Work out the finished part from the listing and answer in its coordinate system (mm). Give positions to 0.01 mm unless a question says otherwise; leave off trailing zeros. Write each loop counter-clockwise with the first axis right and the second up, starting at its lowest first coordinate (ties: lowest second). Pieces come first, ordered by that corner, then holes. Notation, with made-up numbers: (65.5, -24.5) -> (78.5, -24.5) arc R35 cw to (78.5, 14.5) -> close; hole circle Ø6 at (50, 18). An arc over 180 degrees is marked (long way). Use a Markdown table: item, result. Add a question column.
Q1. Consider line 1 (Y direction, x = -174, z = 11.5); line 2 (Y direction, x = 0, z = 12.25); line 3 (Y direction, x = 46.5, z = 1.75). Determine where each line is inside the solid, lowest interval first.
Q2. Section C-C, the plane y = -147.5 is taken. Give the vertices of the cut face in (x, z).
Q3. Each of these flat-tipped pins is pushed along its axis until it touches: pin 1 Ø15 at (x, y) = (174, -174) entering from +Z; pin 2 Ø10 at (x, z) = (-36.5, 16) entering from +Y; pin 3 Ø10 at (x, z) = (-15.5, 12) entering from +Y; pin 4 Ø1.5 at (x, z) = (165.5, 7.5) entering from -Y. Where does it stop, or does it pass through?
Q4. Section D-D, the plane y = -12 is taken. Give the vertices of the cut face in (x, z).
Q5. Section B-B, the plane z = 13.75 is taken. State how many separate pieces and enclosed holes the cut face has, plus the area to 3 significant figures.
Q6. Section A-A, the plane y = 88.5 is taken. Give the vertices of the cut face in (x, z).
from build123d import *

# Parameters (mm, degrees)
F0_R     = 9.5
F0_R_2   = 5
F1_DEPTH = 20


with BuildPart() as f1:
    # F0 (on Top) → F1 (new body)
    with BuildSketch(Plane.XY):
        Polygon((-197, 127), (-167, 127), (-127, 167), (-127, 197), (-197, 197), align=None)
        with Locations((-174, 174)):
            Circle(F0_R, mode=Mode.SUBTRACT)
        Polygon((-167, -127), (-167, 127), (-197, 127), (-197, 30), (-197, -30), (-197, -127), align=None)
        Polygon((-127, 197), (-127, 167), (127, 167), (127, 197), (30, 197), (-30, 197), align=None)
        Polygon((-127, -167), (-167, -127), (-197, -127), (-197, -197), (-127, -197), align=None)
        with Locations((-174, -174)):
            Circle(F0_R, mode=Mode.SUBTRACT)
        Polygon((127, 197), (127, 167), (167, 127), (197, 127), (197, 197), align=None)
        with Locations((174, 174)):
            Circle(F0_R, mode=Mode.SUBTRACT)
        with BuildLine():
            Line((-197, -30), (-197, 30))
            ThreePointArc((-197, 30), (-227, 0), (-197, -30))
        make_face()
        with Locations((-205, 0)):
            Circle(F0_R_2, mode=Mode.SUBTRACT)
        Polygon((127, -167), (-127, -167), (-127, -197), (-30, -197), (30, -197), (127, -197), align=None)
        with BuildLine():
            ThreePointArc((30, 197), (0, 227), (-30, 197))
            Line((-30, 197), (30, 197))
        make_face()
        with Locations((0, 205)):
            Circle(F0_R_2, mode=Mode.SUBTRACT)
        Polygon((197, 127), (167, 127), (167, -127), (197, -127), (197, -30), (197, 30), align=None)
        Polygon((167, -127), (127, -167), (127, -197), (197, -197), (197, -127), align=None)
        with Locations((174, -174)):
            Circle(F0_R, mode=Mode.SUBTRACT)
        with BuildLine():
            Line((30, -197), (-30, -197))
            ThreePointArc((-30, -197), (0, -227), (30, -197))
        make_face()
        with Locations((0, -205)):
            Circle(F0_R_2, mode=Mode.SUBTRACT)
        with BuildLine():
            ThreePointArc((197, -30), (227, 0), (197, 30))
            Line((197, 30), (197, -30))
        make_face()
        with Locations((205, 0)):
            Circle(F0_R_2, mode=Mode.SUBTRACT)
        Polygon((40, 0), (0, -40), (127, -167), (167, -127), align=None)
        Polygon((-40, 0), (-167, -127), (-127, -167), (0, -40), align=None)
        Polygon((-127, 167), (-167, 127), (-40, 0), (0, 40), align=None)
        Polygon((0, 40), (-40, 0), (0, -40), (40, 0), align=None)
        Polygon((167, 127), (127, 167), (0, 40), (40, 0), align=None)
    extrude(amount=F1_DEPTH)


solid = f1.part
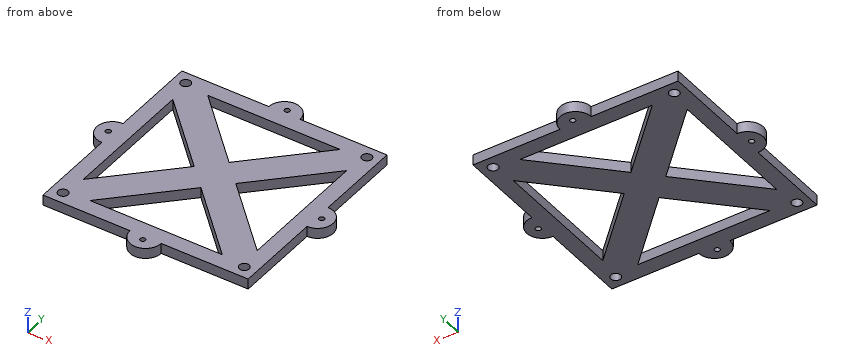
Result set:
| question | item | result |
|---|---|---|
| 1 | line 1 | y = -197 to -183.5, -164.5 to 164.5, 183.5 to 197 |
| 1 | line 2 | y = -227 to -210, -200 to -167, -40 to 40, 167 to 200, 210 to 227 |
| 1 | line 3 | y = -197 to -167, -86.5 to -6.5, 6.5 to 86.5, 167 to 197 |
| 2 | outline | (-197, 0) -> (-107.5, 0) -> (-107.5, 20) -> (-197, 20) -> close; (107.5, 0) -> (197, 0) -> (197, 20) -> (107.5, 20) -> close |
| 3 | pin 1 | passes through |
| 3 | pin 2 | stops at y = 197 |
| 3 | pin 3 | stops at y = 225.1 |
| 3 | pin 4 | stops at y = -197 |
| 4 | outline | (-224.5, 0) -> (-167, 0) -> (-167, 20) -> (-224.5, 20) -> close; (-52, 0) -> (52, 0) -> (52, 20) -> (-52, 20) -> close; (167, 0) -> (224.5, 0) -> (224.5, 20) -> (167, 20) -> close |
| 5 | separate pieces | 1 |
| 5 | enclosed holes | 12 |
| 5 | area | 94,900 mm2 |
| 6 | outline | (-197, 0) -> (-167, 0) -> (-167, 20) -> (-197, 20) -> close; (-128.5, 0) -> (-48.5, 0) -> (-48.5, 20) -> (-128.5, 20) -> close; (48.5, 0) -> (128.5, 0) -> (128.5, 20) -> (48.5, 20) -> close; (167, 0) -> (197, 0) -> (197, 20) -> (167, 20) -> close |
